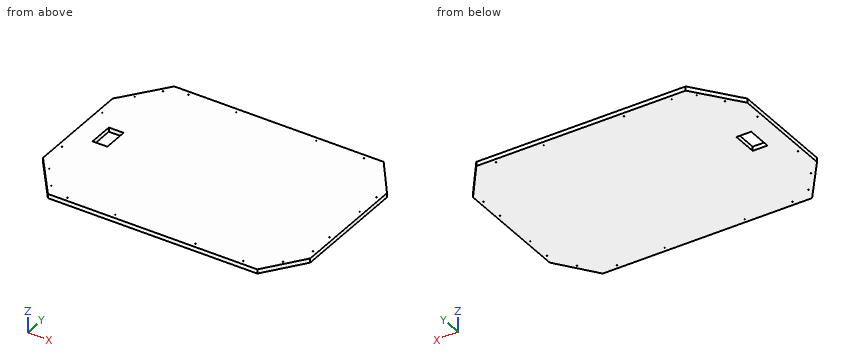
from build123d import *

# Parameters (mm, degrees)
BOSS_EXTRUDE1_DEPTH     = 15
SKETCH9_R               = 1.5
CUT_EXTRUDE1_DEPTH      = 1
CUT_EXTRUDE1_DEPTH_BACK = 16
SKETCH10_W              = 52.6
SKETCH10_H              = 88.9
CUT_EXTRUDE2_DEPTH      = 16


with BuildPart() as part:
    # Sketch2 → Boss-Extrude1 (new body)
    with BuildSketch(Plane.XY):
        Polygon((0, 500.68043587), (118.58, 345.487717935), (863.58, 345.487717935), (963.71, 481.146537036), (963.71, 900.804334703), (863.58, 1036.463153804), (118.58, 1036.463153804), (0, 881.27043587), align=None)
    extrude(amount=BOSS_EXTRUDE1_DEPTH)

    # Sketch9 → Cut-Extrude1 (cut, two sides)
    with BuildSketch(Plane(origin=(0, 0, 0), x_dir=(-1, 0, 0), z_dir=(0, 0, -1))) as cut_extrude1_sk:
        with Locations((-803.58, 1021.463153804)):
            Circle(SKETCH9_R)
        with Locations((-633.58, 1021.463153804)):
            Circle(SKETCH9_R)
        with Locations((-348.58, 1021.463153804)):
            Circle(SKETCH9_R)
        with Locations((-178.58, 1021.463153804)):
            Circle(SKETCH9_R)
        with Locations((-178.58, 360.487717935)):
            Circle(SKETCH9_R)
        with Locations((-348.58, 360.487717935)):
            Circle(SKETCH9_R)
        with Locations((-633.58, 360.487717935)):
            Circle(SKETCH9_R)
        with Locations((-803.58, 360.487717935)):
            Circle(SKETCH9_R)
        with Locations((-905.654330921, 422.269736472)):
            Circle(SKETCH9_R)
        with Locations((-950.019491684, 517.22090145)):
            Circle(SKETCH9_R)
        with Locations((-950.019491684, 864.74090145)):
            Circle(SKETCH9_R)
        with Locations((-950.019491684, 773.32689058)):
            Circle(SKETCH9_R)
        with Locations((-950.019491684, 608.634912319)):
            Circle(SKETCH9_R)
        with BuildLine():
            ThreePointArc((-49.79686308, 923.634087088), (-49.502283169, 925.734854252), (-51.603050333, 926.029434163))
            ThreePointArc((-51.603050333, 926.029434163), (-51.897630244, 923.928666999), (-49.79686308, 923.634087088))
        make_face()
        with BuildLine():
            ThreePointArc((-103.982480668, 995.494499324), (-103.687900757, 997.595266487), (-105.78866792, 997.889846398))
            ThreePointArc((-105.78866792, 997.889846398), (-106.083247831, 995.789079234), (-103.982480668, 995.494499324))
        make_face()
        with BuildLine():
            ThreePointArc((-15.328698966, 802.77043587), (-16.828698966, 801.27043587), (-15.328698966, 799.77043587))
            ThreePointArc((-15.328698966, 799.77043587), (-13.828698966, 801.27043587), (-15.328698966, 802.77043587))
        make_face()
        with BuildLine():
            ThreePointArc((-15.328698966, 582.18043587), (-16.828698966, 580.68043587), (-15.328698966, 579.18043587))
            ThreePointArc((-15.328698966, 579.18043587), (-13.828698966, 580.68043587), (-15.328698966, 582.18043587))
        make_face()
        with BuildLine():
            ThreePointArc((-49.199469581, 459.109041803), (-47.098702418, 459.403621714), (-47.393282329, 461.504388877))
            ThreePointArc((-47.393282329, 461.504388877), (-49.494049492, 461.209808967), (-49.199469581, 459.109041803))
        make_face()
        with BuildLine():
            ThreePointArc((-103.385087169, 387.248629567), (-101.284320005, 387.543209478), (-101.578899916, 389.643976642))
            ThreePointArc((-101.578899916, 389.643976642), (-103.67966708, 389.349396731), (-103.385087169, 387.248629567))
        make_face()
    extrude(amount=CUT_EXTRUDE1_DEPTH, mode=Mode.SUBTRACT)
    extrude(cut_extrude1_sk.sketch, amount=-CUT_EXTRUDE1_DEPTH_BACK, mode=Mode.SUBTRACT)

    # Sketch10 → Cut-Extrude2 (cut, through all)
    with BuildSketch(Plane(origin=(0, 0, 0), x_dir=(-1, 0, 0), z_dir=(0, 0, -1))):
        with Locations((-101.850001448, 699.944225973)):
            Rectangle(SKETCH10_W, SKETCH10_H)
    extrude(amount=-CUT_EXTRUDE2_DEPTH, mode=Mode.SUBTRACT)


solid = part.part
Can you work these out from the model? Positions are in its coordinate system, mm. Round coordinates to 2 decimals unless told otherwise and drop trailing zeros. Use CSV: the item, a comma, the result in double quotes. Start each with the question number.
1) If we section it at A-A on z = 8.75: Count the separate pieces of the cut face and the enclosed holes in it, plus the area to 3 significant figures.
2) For pin 1 Ø2.5 at (x, y) = (15.33, 801.27) entering from -Z; pin 2 Ø7.5 at (x, z) = (100, 5) entering from -Y, each with a flat end and sliding along its axis, tell me the tip position at first contact or that it passes through.
3) Please list where these lines run through material, in increasing order: probe 1 along Y at (x, z) = (178.58, 11.25); probe 2 along X at (y, z) = (689, 1); probe 3 along X at (y, z) = (938, 13.75). Write a range as [from, to].
Geometry results:
1,separate pieces,"1"
1,enclosed holes,"20"
1,area,"629,000 mm2"
2,pin 1,"passes through"
2,pin 2,"stops at y = 364.9"
3,probe 1,"y = [345.49, 358.99], [361.99, 1019.96], [1022.96, 1036.46]"
3,probe 2,"x = [0, 75.55], [128.15, 963.71]"
3,probe 3,"x = [43.35, 936.26]"
